Could you check a few things on this model? Use its own coordinates, in mm. A direction names the side the tool comes from. Coordinates: 2 decimals unless noted, no trailing zeros. Write each loop counter-clockwise with the first axis right and the second up, starting at its lowest first coordinate (ties: lowest second). Pieces come first, ordered by that corner, then holes.
Autodesk Inventor part; units mm, degrees
ref_plane "YZ Plane" through (0, 0, 0) normal (1, 0, 0) x (0, 1, 0)
ref_plane "XZ Plane" through (0, 0, 0) normal (0, 1, 0) x (-1, 0, 0)
ref_plane "XY Plane" through (0, 0, 0) normal (0, 0, 1) x (1, 0, 0)
sketch "Sketch1" plane through (0, 0, 0) normal (0, 0, 1) x (1, 0, 0)
  line L0 (0, 0) -> (88.9, 0)
  line L1 (88.9, 0) -> (88.9, 38.1)
  line L2 (88.9, 38.1) -> (0, 38.1)
  line L3 (0, 38.1) -> (0, 0)
  line L4 (-3.048, 41.148) -> (91.948, 41.148)
  line L5 (91.948, 41.148) -> (91.948, -3.048)
  line L6 (91.948, -3.048) -> (-3.048, -3.048)
  line L7 (-3.048, -3.048) -> (-3.048, 41.148)
  dimension "d0" = 88.9
  dimension "d1" = 38.1
  dimension "d2" = 3.048
extrude "Extrusion1" add sketch "Sketch1" along normal blind 203.2
sketch "Sketch3" plane through (-3.048, 41.148, 0) normal (0, 1, 0) x (1, 0, 0)
  line L0 (0, 0) -> (0, -203.2)
  line L1 (94.996, -203.2) -> (0, -203.2)
  line L2 (15.24, -203.2) -> (17.78, -203.2)
  line L3 (17.78, -203.2) -> (17.78, -177.8)
  line L4 (17.78, -177.8) -> (15.24, -177.8)
  line L5 (15.24, -177.8) -> (15.24, -203.2)
  line L6 (47.498, -203.2) -> (47.498, -149.4712) construction
  line L7 (79.756, -203.2) -> (77.216, -203.2)
  line L8 (77.216, -203.2) -> (77.216, -177.8)
  line L9 (77.216, -177.8) -> (79.756, -177.8)
  line L10 (79.756, -177.8) -> (79.756, -203.2)
  point P0 (3.048, 0)
  dimension "d10" = 2.54
  dimension "d11" = 25.4
  dimension "d12" = 15.24
extrude "Extrusion3" [suppressed]
sketch "Sketch4" plane through (-3.048, 41.148, 0) normal (0, 1, 0) x (1, 0, 0)
  line L0 (94.996, -203.2) -> (0, -203.2)
  line L1 (94.996, -203.2) -> (0, -203.2)
  line L2 (15.24, -177.8) -> (2.54, -177.8)
  line L3 (2.54, -177.8) -> (2.54, -203.2)
  line L4 (2.54, -203.2) -> (15.24, -203.2)
  line L5 (15.24, -203.2) -> (15.24, -177.8)
  line L6 (47.498, -203.2) -> (47.498, -154.3799) construction
  line L7 (79.756, -203.2) -> (79.756, -177.8)
  line L8 (79.756, -177.8) -> (92.456, -177.8)
  line L9 (92.456, -177.8) -> (92.456, -203.2)
  line L10 (92.456, -203.2) -> (79.756, -203.2)
  line L11 (79.756, -203.2) -> (79.756, -177.8)
  point P0 (17.78, -203.2)
  point P1 (77.216, -203.2)
  point P2 (15.24, -203.2)
  point P3 (3.048, 0)
  dimension "d15" = 12.7
extrude "Extrusion4" [suppressed]
sketch "Sketch5" plane through (0, 0, 0) normal (0, 1, 0) x (1, 0, 0)
  line L0 (0, 0) -> (0, -203.2)
  line L1 (88.9, -203.2) -> (0, -203.2)
  line L2 (31.75, -161.29) -> (57.15, -161.29)
  line L3 (57.15, -161.29) -> (57.15, -158.75)
  line L4 (57.15, -158.75) -> (31.75, -158.75)
  line L5 (31.75, -158.75) -> (31.75, -161.29)
  dimension "d18" = 25.4
  dimension "d19" = 31.75
  dimension "d20" = 44.45
  dimension "d21" = 2.54
extrude "Extrusion5" add sketch "Sketch5" along normal blind 12.7
sketch "Sketch6" plane through (0, 0, 0) normal (0, 1, 0) x (1, 0, 0)
  line L0 (31.75, -158.75) -> (57.15, -158.75)
  line L1 (57.15, -158.75) -> (57.15, -146.05)
  line L2 (57.15, -146.05) -> (31.75, -146.05)
  line L3 (31.75, -146.05) -> (31.75, -158.75)
  dimension "d24" = 25.4
  dimension "d25" = 12.7
extrude "Extrusion6" cut sketch "Sketch6" against normal blind 12.7
sketch "Sketch7" plane through (12.192, 38.1, 203.2) normal (-1, 0, 0) x (0, 0, 1)
  line L0 (-25.4, 15.748) -> (0, 15.748)
  circle A0 centre (-12.7, 10.668) radius 0.6717
  point P0 (-203.2, -38.1)
  dimension "d28" = 5.08
hole "Hole1" [suppressed]
sketch "Sketch11" plane through (-3.048, 41.148, 0) normal (0, 1, 0) x (1, 0, 0)
  line L0 (0, 0) -> (94.996, 0)
  line L1 (94.996, -203.2) -> (0, -203.2)
  line L2 (47.498, 0) -> (47.498, -203.2) construction
  line L3 (34.798, -196.85) -> (60.198, -196.85)
  line L4 (60.198, -196.85) -> (60.198, -165.1)
  line L5 (60.198, -165.1) -> (34.798, -165.1)
  line L6 (34.798, -165.1) -> (34.798, -196.85)
  point P0 (3.048, 0)
  dimension "d60" = 6.35
  dimension "d61" = 31.75
  dimension "d62" = 25.4
extrude "Extrusion8" cut sketch "Sketch11" against normal blind 12.7
sketch "Sketch12" plane through (-3.048, 41.148, 0) normal (0, 1, 0) x (1, 0, 0)
  line L0 (0, 0) -> (94.996, 0)
  line L1 (0, 0) -> (0, -203.2)
  circle A0 centre (22.098, -19.05) radius 3.175
  circle A1 centre (72.898, -19.05) radius 3.175
  point P0 (3.048, 0)
  dimension "d65" = 6.35
  dimension "d66" = 19.05
  dimension "d67" = 22.098
  dimension "d68" = 6.35
  dimension "d70" = 50.8
hole "Hole3" at (19.05, 41.148, 19.05) at (69.85, 41.148, 19.05) direction (0, -1, 0) diameter 6.35 depth 25.4 tip angle 118
sketch "Sketch13" plane through (-3.048, 41.148, 0) normal (0, 1, 0) x (1, 0, 0)
  circle A0 centre (22.098, -19.05) radius 3.175
  circle A1 centre (72.898, -19.05) radius 3.175
  line L0 (94.996, 0) -> (94.996, -203.2)
  line L1 (22.098, -19.05) -> (72.898, -19.05) construction
  circle A2 centre (47.498, -57.15) radius 3.5871
  point P0 (3.048, 0)
  dimension "d80" = 38.1
hole "Hole4" at (44.45, 41.148, 57.15) direction (0, -1, 0) diameter 6.35 end through all
properties part number "2p1h37" material "Steel, Galvanized"
1. I want a section at D-D on x = 19.05. Please give me the cut outline in (y, z) (3 decimals), plus the area to 3 significant figures.
Verdict:
outline: (-3.048, 0) - (0, 0) - (0, 203.2) - (-3.048, 203.2) - close; (38.1, 0) - (41.148, 0) - (41.148, 15.875) - (38.1, 15.875) - close; (38.1, 22.225) - (41.148, 22.225) - (41.148, 203.2) - (38.1, 203.2) - close
area: 1,220 mm2
2. I want a section at C-C on z = 57.15. Please give me the cut outline in (x, y) (3 decimals), plus the area to 3 significant figures.
Verdict:
outline: (-3.048, -3.048) - (41.275, -3.048) - (41.275, 0) - (0, 0) - (0, 38.1) - (41.275, 38.1) - (41.275, 41.148) - (-3.048, 41.148) - close; (47.625, -3.048) - (91.948, -3.048) - (91.948, 41.148) - (47.625, 41.148) - (47.625, 38.1) - (88.9, 38.1) - (88.9, 0) - (47.625, 0) - close
area: 773 mm2
3. If we mould it in two halves opening along Y, with no side actions, what happens to faces 6 (the face through (42.304, -1.545, 54.81)), 7 (the face through (45, -3.048, 100)), 8 (the face through (0, 19, 100))? For each: pulls with the +Y half, pulls with the -Y half, needs draft (parallel to the pull), parting line crosses it, or undercut.
Verdict:
face 6: needs draft
face 7: pulls with the -Y half
face 8: undercut
4. For pin 1 (12 mm diameter, centred on x = 25, y = 6.5, fed in from -Z); pin 2 (5 mm diameter, centred on x = 19.05, z = 19.05, fed in from +Y); pin 3 (2.5 mm diameter, centred on x = 39.5, y = 39, fed in from -Z), each with a flat end and sliding along its axis, tell me the tip position at first contact or that it passes through.
Verdict:
pin 1: passes through
pin 2: stops at y = 0
pin 3: stops at z = 0
5. On a 3-axis mill with a long thin cutter (end or side, diameter ignored), from which of +Z, -Z, +X, -X, +Y, -Y can I reach the whole of each face in a straight line? I mean faces 1 (the face through (40.7, -0.5, 0)), 2 (the face through (45, 38.1, 100)), 3 (the face through (72.95, 39.6, 18.36)), 4 (the face through (44, 6, 161.29)), 5 (the face through (44, 5, 158.75)). Say none if no direction works.
Verdict:
face 1: -Z, +X, -X, +Y, -Y
face 2: +Z, -Z
face 3: +Y
face 4: +Z
face 5: -Y
6. I want a section at A-A on x = 84. Please give me the cut outline in (y, z).
Verdict:
outline: (-3.05, 0) - (0, 0) - (0, 203.2) - (-3.05, 203.2) - close; (38.1, 0) - (41.15, 0) - (41.15, 203.2) - (38.1, 203.2) - close
7. I want a section at B-B on y = 29. Please give me the cut outline in (x, z).
Verdict:
outline: (-3.05, 0) - (0, 0) - (0, 203.2) - (-3.05, 203.2) - close; (88.9, 0) - (91.95, 0) - (91.95, 203.2) - (88.9, 203.2) - close
8. Please list where these lines run through material, in increasing order: line 1 along X through (y, z) = (39, 19); line 2 along Z through (x, y) = (44, 39); line 3 along Y through (x, z) = (43, 50.5).
Verdict:
line 1: x = -3.05 to 15.88, 22.22 to 66.68, 73.02 to 91.95
line 2: z = 0 to 54.01, 60.29 to 165.1, 196.85 to 203.2
line 3: y = -3.05 to 0, 38.1 to 41.15
